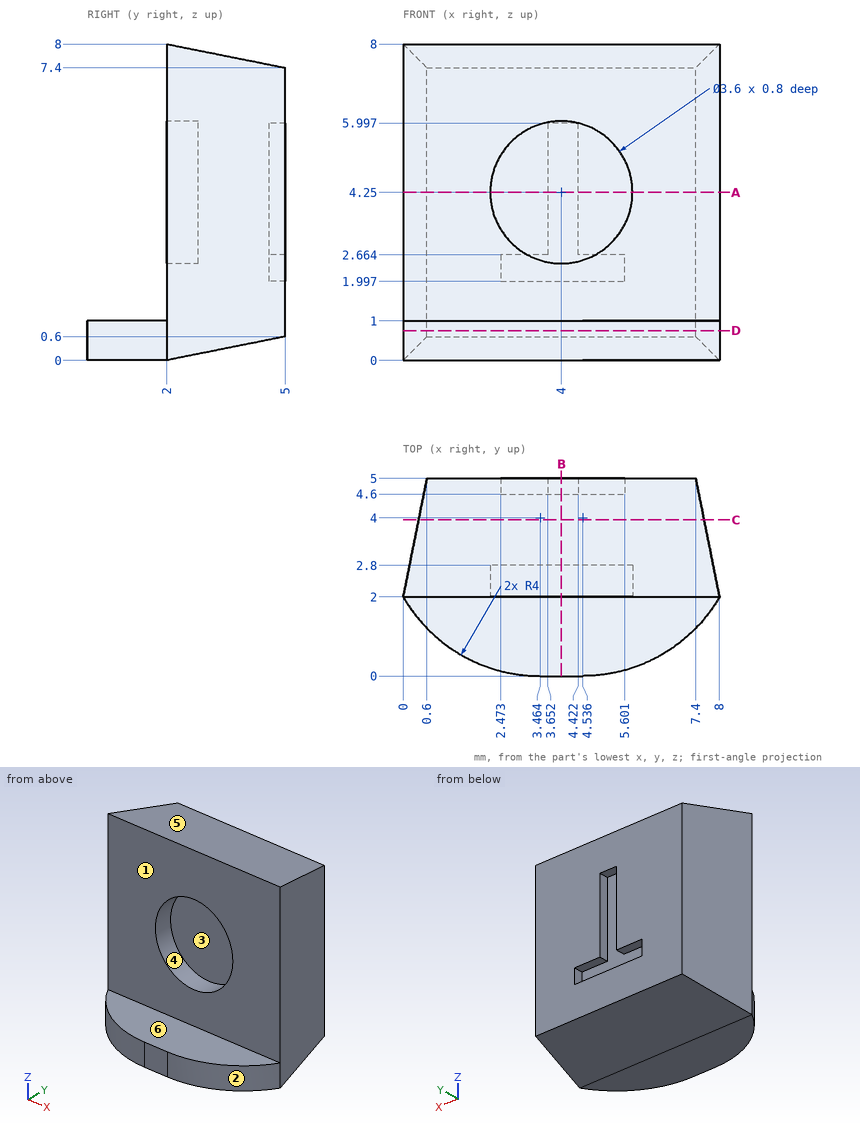
Study the drawing (mm; zero at the part's minimum x, y, z) and answer. A direction names the side the tool comes from. Coordinates: 2 decimals unless noted, no trailing zeros. Order: outer loops, then holes, each group sorted by start corner. A loop starts at its lowest first (then second) coordinate and runs counter-clockwise, first axis right, second up. Notation, with made-up numbers: M 50,63 L 72,63 A22 ccw 72,95 Z; hole C 72.25,36.25 d8. An arc over 180 degrees is marked long. Answer as a JSON object with one key per item and string values. Group by question number.
1. A tool of negligible diameter and unlimited length cuts with its end or side. For the marked faces 4, 5 and 6, from which of +Z, -Z, +X, -X, +Y, -Y can it reach the whole face along a straight path? Write none if from no direction.
2. Section A-A on z = 4.25 is taken. Write down the section's boundary in (x, y), then the cut area to 3 significant figures.
3. Straight lines are drawn through the part: line 1 (Y direction, x = 4.5, z = 2.25); line 2 (Y direction, x = 1, z = 2.5); line 3 (X direction, y = 2.3, z = 4.25). For each, find the intervals that lie inside material, in ascending order.
4. Determine the mould class of the marked faces 1, 2 and 3 for opening direction X: released by +X, released by -X, zero draft, split by the parting line, or undercut.
5. Flat-ended cylindrical pins translate along their axes: P1, Ø1.6, axis at x = 2, y = 1, coming from the +Z side; P2, Ø3, axis at x = 4, z = 4.5, coming from the -Y side; P3, Ø3.5, axis at x = 5.5, z = 5.5, coming from the -Y side. Find the tip coordinate at first contact, or state that the pin passes through.
6. Section D-D on z = 0.75 is taken. Write down the section's boundary in (x, y), then the cut area to 3 significant figures.
7. Section C-C on y = 3.95 is taken. Write down the section's boundary in (x, z).
8. Section B-B on x = 4 is taken. Write down the section's boundary in (y, z).
Values follow:
{
 "1": {"face 4": "-Y", "face 5": "+Z, +X, -X, +Y", "face 6": "+Z, +X, -X, -Y"},
 "2": {"outline": "M 0,2 L 2.2,2 L 2.2,2.8 L 5.8,2.8 L 5.8,2 L 8,2 L 7.4,5 L 4.42,5 L 4.42,4.6 L 3.65,4.6 L 3.65,5 L 0.6,5 Z", "area": "19.0 mm2"},
 "3": {"line 1": "2 to 4.6", "line 2": "2 to 5", "line 3": "0.06 to 2.2, 5.8 to 7.94"},
 "4": {"face 1": "zero draft", "face 2": "released by +X", "face 3": "undercut"},
 "5": {"P1": "z = 1", "P2": "y = 2.8", "P3": "y = 2"},
 "6": {"outline": "M 0,2 A4 ccw 3.46,0 L 4.54,0 A4 ccw 8,2 L 7.4,5 L 0.6,5 Z", "area": "34.2 mm2"},
 "7": {"outline": "M 0.39,0.39 L 7.61,0.39 L 7.61,7.61 L 0.39,7.61 Z"},
 "8": {"outline": "M 0,0 L 2,0 L 5,0.6 L 5,2 L 4.6,2 L 4.6,6 L 5,6 L 5,7.4 L 2,8 L 2,6.05 L 2.8,6.05 L 2.8,2.45 L 2,2.45 L 2,1 L 0,1 Z"}
}
